Work out the finished part from the listing and answer in its coordinate system (mm). Face numbers are marked on the shaded views. A direction names the side the tool comes from. Coordinates: 2 decimals unless noted, no trailing zeros. Order: outer loops, then holes, each group sorted by start corner. A loop starts at its lowest first (then second) coordinate and runs counter-clockwise, first axis right, second up.
1. The part is cut by section A-A, the plane z = 0. Give the vertices of the cut face in (x, y), then the cut area to 3 significant figures.
2. Find the intervals of material crossed by probe 1 along X at (y, z) = (-1.5, -2.25); probe 2 along Z at (x, y) = (14.5, 0); probe 3 along X at (y, z) = (0.5, -2.25), in increasing order.
3. The part is cut by section C-C, the plane x = 7.75. Give the vertices of the cut face in (y, z), then the cut area to 3 significant figures.
4. The part is cut by section B-B, the plane y = 0. Give the vertices of the cut face in (x, z), then the cut area to 3 significant figures.
5. Flat-ended cylindrical pins translate along their axes: pin 1 Ø1 at (y, z) = (3, -3) entering from +X; pin 2 Ø3 at (x, z) = (17, -2.5) entering from +Y; pin 3 Ø1.1 at (x, z) = (0.5, -1.5) entering from +Y. Find the tip coordinate at first contact, or state that the pin passes through.
6. A tool of negligible diameter and unlimited length cuts with its end or side. For the marked faces 1 and 2, from which of +Z, -Z, +X, -X, +Y, -Y can it reach the whole face along a straight path? Write none if from no direction.
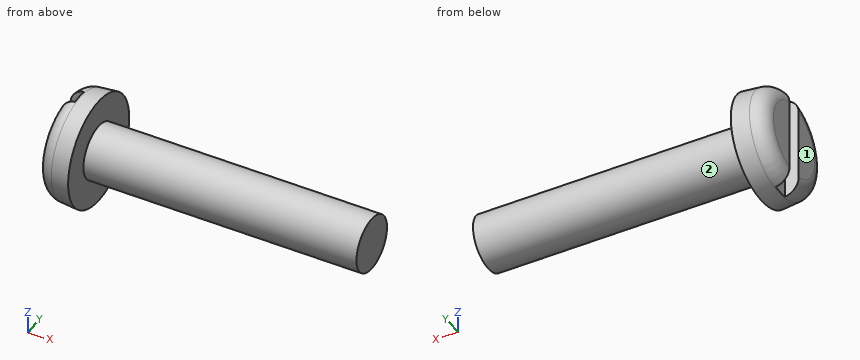
```python
from build123d import *

# Parameters (mm, degrees)
FILLET2_R  = 1.2
SKETCH2_W  = 8
SKETCH2_H  = 1.2
SLOT_DEPTH = 1


with BuildPart() as part:
    # BodySke → Base-Revolve (revolve)
    with BuildSketch(Plane.XY):
        Polygon((2.4, 2), (2.4, 4), (0, 3.790027208), (0, 0), (22.4, 0), (22.4, 2), align=None)
    revolve(axis=Axis((-25.4, 0, 0), (1, 0, 0)))

    # Fillet2
    fillet2_edges = [part.edges().sort_by_distance(p)[0] for p in [
        (0, -3.790027208, 0),
    ]]
    fillet(fillet2_edges, radius=FILLET2_R)

    # Sketch2 → Slot (cut)
    with BuildSketch(Plane(origin=(0, 0, 0), x_dir=(0, 0, -1), z_dir=(1, 0, 0))):
        Rectangle(SKETCH2_W, SKETCH2_H)
    extrude(amount=SLOT_DEPTH, mode=Mode.SUBTRACT)


solid = part.part
```
Geometry says:
1. outline: (0, -2.69) arc R1.2 ccw to (1.1, -3.89) - (2.4, -4) - (2.4, -2) - (22.4, -2) - (22.4, 2) - (2.4, 2) - (2.4, 4) - (1.1, 3.89) arc R1.2 ccw to (0, 2.69) - (0, 0.6) - (1, 0.6) - (1, -0.6) - (0, -0.6) - close
1. area: 97.0 mm2
2. probe 1: x = 0 to 2.4
2. probe 2: z = -2 to 2
2. probe 3: x = 1 to 2.4
3. outline: circle Ø4 at (0, 0)
3. area: 12.6 mm2
4. outline: (1, -3.87) arc R1.2 ccw to (1.1, -3.89) - (2.4, -4) - (2.4, -2) - (22.4, -2) - (22.4, 2) - (2.4, 2) - (2.4, 4) - (1.1, 3.89) arc R1.2 ccw to (1, 3.87) - close
4. area: 91.0 mm2
5. pin 1: stops at x = 2.4
5. pin 2: stops at y = 1.73
5. pin 3: stops at y = 3.69
6. face 1: +Z, -Z, -X, +Y, -Y
6. face 2: +X
